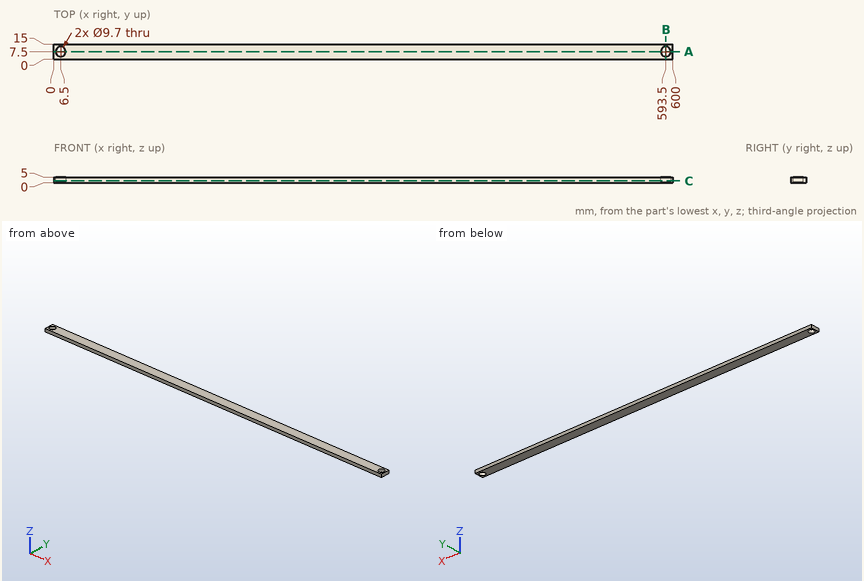
Could you check a few things on this drawing? It's one solid part, dimensions in mm from its lowest x, y, z. Give positions to 0.01 mm unless a question says otherwise; leave off trailing zeros. Loops run counter-clockwise (first coordinate to the right, second up) from the corner with the lowest first, then second, coordinate; pieces in that order, holes last. Notation, with made-up numbers: M 41,25 L 88,25 A18 ccw 88,51 Z; hole C 33,74.5 d11. An arc over 180 degrees is marked long. Return JSON: item names as keys, results as strings.
Item 1: Imagine slicing it at B-B on x = 593.5. List the corners of the cut face in (y, z) for me.
A:
{"outline": "M 0,0 L 2.65,0 L 2.65,5 L 0,5 Z; M 12.35,0 L 15,0 L 15,5 L 12.35,5 Z"}
Item 2: Imagine slicing it at A-A on y = 7.5. List the corners of the cut face in (x, z) for me.
A:
{"outline": "M 0,0 L 1.65,0 L 1.65,5 L 0,5 Z; M 11.35,0 L 588.65,0 L 588.65,5 L 11.35,5 Z; M 598.35,0 L 600,0 L 600,5 L 598.35,5 Z"}
Item 3: Imagine slicing it at C-C on z = 1.75. List the corners of the cut face in (x, y) for me.
A:
{"outline": "M 0,0 L 600,0 L 600,15 L 0,15 Z; hole C 6.5,7.5 d9.7; hole C 593.5,7.5 d9.7"}
Item 4: Please list where these lines run through material, in increasing order: line 1 (X direction, y = 7, z = 2.7); line 2 (Y direction, x = 6.5, z = 1.85); line 3 (X direction, y = 3.5, z = 2).
A:
{"line 1": "x = 0 to 1.68, 11.32 to 588.68, 598.32 to 600", "line 2": "y = 0 to 2.65, 12.35 to 15", "line 3": "x = 0 to 3.76, 9.24 to 590.76, 596.24 to 600"}
